from build123d import *

# Parameters (mm, degrees)
SKETCH1_R                = 14.5
SKETCH1_R_2              = 12.5
BOSS_EXTRUDE1_DEPTH      = 25
BOSS_EXTRUDE2_DEPTH      = 14.5
BOSS_EXTRUDE2_DEPTH_BACK = 14.5
SKETCH3_R                = 5.997794038
CUT_EXTRUDE1_DEPTH       = 25
SKETCH4_W                = 10
SKETCH4_H                = 3
CUT_EXTRUDE2_DEPTH       = 30
SKETCH6_R                = 1.5
CUT_EXTRUDE4_DEPTH       = 30


with BuildPart() as part:
    # Sketch1 → Boss-Extrude1 (new body)
    with BuildSketch(Plane(origin=(0, 0, 0), x_dir=(1, 0, 0), z_dir=(0, 1, 0))):
        with Locations(Location((0, 0, 0), (0, 0, 270))):
            Circle(SKETCH1_R)
        with Locations(Location((0, 0, 0), (0, 0, 270))):
            Circle(SKETCH1_R_2, mode=Mode.SUBTRACT)
    extrude(amount=BOSS_EXTRUDE1_DEPTH)

    # Sketch2 → Boss-Extrude2 (add, two sides: drawn at the far end of the back side and taken through both)
    with BuildSketch(Plane.XY.offset(-BOSS_EXTRUDE2_DEPTH_BACK)):
        with BuildLine():
            Line((-11.25, -11.25), (-20, -11.25))
            Line((-20, -11.25), (-24, -11.25))
            Line((-24, -11.25), (-24, -8.25))
            Line((-24, -8.25), (-20, -8.25))
            Line((-20, -8.25), (-15.002024714, -8.25))
            ThreePointArc((-15.002024714, -8.25), (-14.270980746, -7.932330358), (-14.004397729, -7.181149435))
            Line((-14.004397729, -7.181149435), (-14.5, 0))
            Line((-14.5, 0), (-8.746427842, 0))
            ThreePointArc((-8.746427842, 0), (0, 3), (8.746427842, 0))
            Line((8.746427842, 0), (14.5, 0))
            Line((14.5, 0), (14.004397729, -7.181149435))
            ThreePointArc((14.004397729, -7.181149435), (14.270980746, -7.932330358), (15.002024714, -8.25))
            Line((15.002024714, -8.25), (20, -8.25))
            Line((20, -8.25), (24, -8.25))
            Line((24, -8.25), (24, -11.25))
            Line((24, -11.25), (20, -11.25))
            Line((20, -11.25), (11.25, -11.25))
            ThreePointArc((11.25, -11.25), (0, 0), (-11.25, -11.25))
        make_face()
    extrude(amount=BOSS_EXTRUDE2_DEPTH + BOSS_EXTRUDE2_DEPTH_BACK)

    # Sketch3 → Cut-Extrude1 (cut)
    with BuildSketch(Plane.XZ.offset(11.25)):
        with Locations(Location((0, 0, 0), (0, 0, 270))):
            Circle(SKETCH3_R)
    extrude(amount=-CUT_EXTRUDE1_DEPTH, mode=Mode.SUBTRACT)

    # Sketch4 → Cut-Extrude2 (cut)
    with BuildSketch(Plane(origin=(0, 0, -14.5), x_dir=(-1, 0, 0), z_dir=(0, 0, -1))):
        with Locations((0, 6.23565899)):
            Rectangle(SKETCH4_W, SKETCH4_H)
    extrude(amount=-CUT_EXTRUDE2_DEPTH, mode=Mode.SUBTRACT)

    # Sketch6 → Cut-Extrude4 (cut)
    with BuildSketch(Plane(origin=(0, -8.25, 0), x_dir=(1, 0, 0), z_dir=(0, 1, 0))):
        with Locations(Location((-19.501012357, 0, 0), (0, 0, 270))):
            Circle(SKETCH6_R)
        with Locations(Location((19.501012357, 0, 0), (0, 0, 270))):
            Circle(SKETCH6_R)
    extrude(amount=-CUT_EXTRUDE4_DEPTH, mode=Mode.SUBTRACT)


solid = part.part
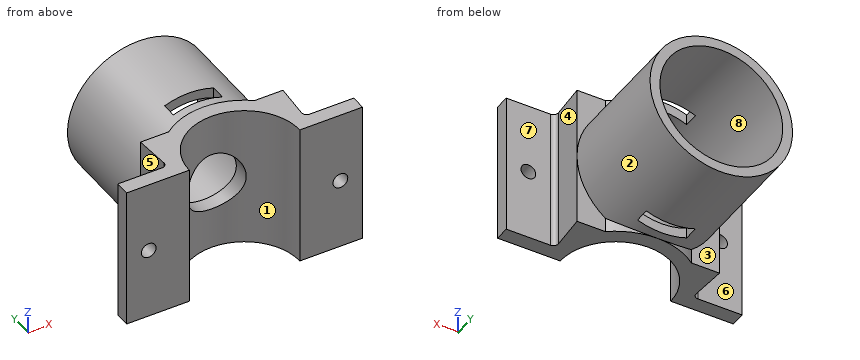
Source: CAD feature listing. Evaluate the final solid. Frame: model axes, mm. Face numbers are marked on the shaded views. A direction names the side the tool comes from. Give positions to 0.01 mm unless a question says otherwise; leave off trailing zeros. Write each loop counter-clockwise with the first axis right and the second up, starting at its lowest first coordinate (ties: lowest second). Pieces come first, ordered by that corner, then holes. Notation, with made-up numbers: (-14, 33) -> (-6, 33) arc R19 cw to (-6, 65) -> close; hole circle Ø6 at (47.5, 3.5). An arc over 180 degrees is marked (long way). Write item = value, one per line.
Q1. Reachability of the marked faces 4, 5, 6, 7 and 8 from +Z, -Z, +X, -X, +Y, -Y: full face, straight path, thin tool, end or side. Return the list, or none.
Here are the results:
face_4 = +Z, -Z, +X
face_5 = +Z, -Z, -X
face_6 = +Z, -Z, -X, +Y
face_7 = +Z, -Z, +X, +Y
face_8 = +Y
Q2. Cut plane D-D on z = -10.5. Return loops of the section in (x, y), then the cut area to 3 significant figures.
Here are the results:
outline = (-24, -11.25) -> (-11.25, -11.25) arc R11.25 cw to (11.25, -11.25) -> (24, -11.25) -> (24, -8.25) -> (15, -8.25) arc R1 cw to (14, -7.18) -> (14.5, 0) -> (10, 0) -> (10, 25) -> (6.78, 25) -> (6.78, 1.28) arc R14.25 ccw to (-6.78, 1.28) -> (-6.78, 25) -> (-10, 25) -> (-10, 0) -> (-14.5, 0) -> (-14, -7.18) arc R1 cw to (-15, -8.25) -> (-24, -8.25) -> close
area = 374 mm²
Q3. Cut plane B-B on z = -2.5. Return loops of the section in (x, y).
Here are the results:
outline = (-24, -11.25) -> (-11.25, -11.25) arc R11.25 cw to (-5.45, -1.41) -> (-5.45, 1.92) arc R14.25 ccw to (-8.75, 0) -> (-12.25, 0) -> (-12.25, 25) -> (-14.28, 25) -> (-14.28, 0) -> (-14.5, 0) -> (-14, -7.18) arc R1 cw to (-15, -8.25) -> (-24, -8.25) -> close; (5.45, -1.41) arc R11.25 cw to (11.25, -11.25) -> (24, -11.25) -> (24, -8.25) -> (15, -8.25) arc R1 cw to (14, -7.18) -> (14.5, 0) -> (14.28, 0) -> (14.28, 25) -> (12.25, 25) -> (12.25, 0) -> (8.75, 0) arc R14.25 ccw to (5.45, 1.92) -> close
Q4. Mould query, pull axis X, two halves, no side actions, for the marked faces 1, 2 and 3. Classes: +X half, -X half, draft (parallel to the pull), parting line (faces both ways), or undercut.
Here are the results:
face_1 = undercut
face_2 = parting line
face_3 = draft
Q5. First-contact query: pin 1 (5 mm diameter, centred on x = -15.5, z = 7.5, fed in from +Y); pin 2 (1 mm diameter, centred on y = 13.5, z = 4, fed in from -X); pin 3 (3.5 mm diameter, centred on x = -1, z = -13.5, fed in from -Y); pin 4 (3 mm diameter, centred on x = 11.5, z = -9.5, fed in from +Y). Flat tips, straight axial feed; report the tip coordinate or a pass-through.
Here are the results:
pin_1 = 0
pin_2 = -14.07
pin_3 = -0.34
pin_4 = 25
Q6. Cut plane A-A on y = 7. Return loops of the section in (x, z).
Here are the results:
outline = (-5, -13.61) -> (-5, -11.46) arc R12.5 cw to (-5, 11.46) -> (-5, 13.61) arc R14.5 ccw to start; (5, -13.61) arc R14.5 ccw to (5, 13.61) -> (5, 11.46) arc R12.5 cw to (5, -11.46) -> close
Q7. Line query: line 1 (X direction, y = -10.45, z = 0); line 2 (Y direction, x = 19, z = -7); line 3 (X direction, y = 1, z = 7.25). Output: solid intervals per line, ascending. Write a range as from..to.
Here are the results:
line_1 = -24..-21, -18..-11.22, 11.22..18, 21..24
line_2 = -11.25..-8.25
line_3 = -12.56..-10.18, -7.28..7.28, 10.18..12.56
Q8. Cut plane C-C on y = -3. Return loops of the section in (x, z), then the cut area to 3 significant figures.
Here are the results:
outline = (-14.29, -14.5) -> (-7.65, -14.5) -> (-7.65, 14.5) -> (-14.29, 14.5) -> close; (7.65, -14.5) -> (14.29, -14.5) -> (14.29, 14.5) -> (7.65, 14.5) -> close
area = 385 mm²
